Geometry: final body of the model. Coordinates: model frame, mm. A direction names the side the tool comes from. Give positions to 0.01 mm unless a question says otherwise; leave off trailing zeros. Write each loop counter-clockwise with the first axis right and the second up, starting at its lowest first coordinate (ties: lowest second). Pieces come first, ordered by that corner, then holes.
```python
from build123d import *

# Parameters (mm, degrees)
F0_W     = 30
F0_H     = 10
F1_DEPTH = 20
F2_R     = 2.1
F3_DEPTH = 10
F4_W     = 26.5
F4_H     = 1.2
F5_DEPTH = 10
F6_R     = 3.75
F7_DEPTH = 4.5


with BuildPart() as f1:
    # F0 (on Top) → F1 (new body)
    with BuildSketch(Plane.XY):
        Rectangle(F0_W, F0_H)
    extrude(amount=F1_DEPTH)

    # F2 (on face) → F3 (cut, through all)
    with BuildSketch(Plane.XZ.offset(5)):
        with Locations((0, 6)):
            Circle(F2_R)
    extrude(amount=-F3_DEPTH, mode=Mode.SUBTRACT)

    # F4 (on face) → F5 (cut)
    with BuildSketch(Plane.XY.offset(20)):
        with Locations((0, 3.1)):
            Rectangle(F4_W, F4_H)
        with Locations((0, -3.1)):
            Rectangle(F4_W, F4_H)
    extrude(amount=-F5_DEPTH, mode=Mode.SUBTRACT)

    # F6 (on face) → F7 (cut)
    with BuildSketch(Plane.XZ.offset(5)):
        with Locations((0, 6)):
            Circle(F6_R)
    extrude(amount=-F7_DEPTH, mode=Mode.SUBTRACT)


solid = f1.part
```
Item 1: Pin query (flat end, axial travel): pin 1 Ø6 at (x, z) = (-0.5, 6) entering from -Y. Return the tip coordinate at first contact, or that it passes through.
Found:
pin 1: stops at y = -0.5
Item 2: Pull-direction query (Y, two-part tool) for faces 4 (the face through (-13.25, -3, 15)), 5 (the face through (0, -5, 10)), 6 (the face through (0, -2.5, 15)), 7 (the face through (0, 0, 0)); classes: +Y half, -Y half, draft (parallel to the pull), parting line (faces both ways), or undercut.
Found:
face 4: undercut
face 5: -Y half
face 6: undercut
face 7: draft
Item 3: Reachability of faces 1 (the face through (0, -3.7, 15)), 2 (the face through (0, 0, 20)), 3 (the face through (-0.81, -2.78, 2.34)) from +Z, -Z, +X, -X, +Y, -Y: full face, straight path, thin tool, end or side. Return the list, or none.
Found:
face 1: +Z
face 2: +Z, +X, -X, +Y, -Y
face 3: -Y
Item 4: Section D-D, the plane z = 17.25. Return the cut outline in (x, y), plus the area to 3 significant figures.
Found:
outline: (-15, -5) - (15, -5) - (15, 5) - (-15, 5) - close; hole (-13.25, -3.7) - (13.25, -3.7) - (13.25, -2.5) - (-13.25, -2.5) - close; hole (-13.25, 2.5) - (13.25, 2.5) - (13.25, 3.7) - (-13.25, 3.7) - close
area: 236 mm2
Item 5: Section A-A, the plane z = 6. Return the cut outline in (x, y), plus the area to 3 significant figures.
Found:
outline: (-15, -5) - (-3.75, -5) - (-3.75, -0.5) - (-2.1, -0.5) - (-2.1, 5) - (-15, 5) - close; (2.1, -0.5) - (3.75, -0.5) - (3.75, -5) - (15, -5) - (15, 5) - (2.1, 5) - close
area: 243 mm2
Item 6: Section C-C, the plane y = -1.75. Return the cut outline in (x, z), plus the area to 3 significant figures.
Found:
outline: (-15, 0) - (15, 0) - (15, 20) - (-15, 20) - close; hole circle Ø7.5 at (0, 6)
area: 556 mm2
Item 7: Section B-B, the plane x = 0. Return the cut outline in (y, z).
Found:
outline: (-5, 0) - (5, 0) - (5, 3.9) - (-0.5, 3.9) - (-0.5, 2.25) - (-5, 2.25) - close; (-5, 9.75) - (-0.5, 9.75) - (-0.5, 8.1) - (5, 8.1) - (5, 20) - (3.7, 20) - (3.7, 10) - (2.5, 10) - (2.5, 20) - (-2.5, 20) - (-2.5, 10) - (-3.7, 10) - (-3.7, 20) - (-5, 20) - close
Item 8: Line query: L1, parallel to Y at x = -11.75, z = 18.5; L2, parallel to X at y = -3, z = 12; L3, parallel to Z at x = 0, y = -1.6. Output: solid intervals per line, ascending.
Found:
L1: y = -5 to -3.7, -2.5 to 2.5, 3.7 to 5
L2: x = -15 to -13.25, 13.25 to 15
L3: z = 0 to 2.25, 9.75 to 20
